from build123d import *

# Parameters (mm, degrees)
SKETCH_W     = 40
SKETCH_H     = 20
PAD_DEPTH    = 2
SKETCH001_W  = 40
SKETCH001_H  = 2.5
PAD001_DEPTH = 10


with BuildPart() as part:
    # Sketch → Pad (new body)
    with BuildSketch(Plane.XY):
        with Locations((20, 10)):
            Rectangle(SKETCH_W, SKETCH_H)
    extrude(amount=PAD_DEPTH)

    # Sketch001 (on Face6 of Pad) → Pad001 (join)
    with BuildSketch(Plane.XY.offset(2)):
        with Locations((20, 1.25)):
            Rectangle(SKETCH001_W, SKETCH001_H)
        with Locations((20, 18.75)):
            Rectangle(SKETCH001_W, SKETCH001_H)
        Polygon((0, 2.5), (0, 0), align=None)
    extrude(amount=PAD001_DEPTH)


solid = part.part
Build history of the part. All positions in model axes, mm. A direction names the side the tool comes from. Round coordinates to 2 decimals unless told otherwise and drop trailing zeros. Write each loop counter-clockwise with the first axis right and the second up, starting at its lowest first coordinate (ties: lowest second). Pieces come first, ordered by that corner, then holes. Notation, with made-up numbers: M -26.75,-8 L 16.25,-8 A17 cw 16.25,-1 Z; hole C -39,-22 d8. An arc over 180 degrees is marked long. Answer as a JSON object with one key per item and string values. Group by question number.
(1) Cut at B-B (x = 29). Give the cut face in (y, z).
(2) Drill centre lines: L1, parallel to Y at x = 37, z = 11; L2, parallel to Z at x = 18.5, y = 8.5. Where is each one in solid material? Low to high.
(3) Cut at A-A (z = 6.5). Give the cut face in (x, y), and give its area (3 significant figures).
(4) Cut at C-C (y = 12.5). Give the cut face in (x, z).
(5) Which spindle directions (+Z, -Z, +X, -X, +Y, -Y) get a long thin tool onto all of the face, cutting with end or side? Do faces 1 (the flat face through (20, 10, 0)), 2 (the flat face through (20, 2.5, 7)). Say none if no direction does.
(6) Mould opens along Y. For faces 3 (the flat face through (20, 17.5, 7)), 4 (the flat face through (20, 1, 12)), 5 (the flat face through (20, 20, 6)) say: pulls with the +Y half, pulls with the -Y half, needs draft (parallel to the pull), parting line crosses it, or undercut.
(7) Flat gauge pin, fed straight in: pin 1 (7.5 mm diameter, centred on x = 28, y = 12.5, fed in from +Z). Where does the tip first touch, or does it go through?
Responses:
{
 "1": {"outline": "M 0,0 L 20,0 L 20,12 L 17.5,12 L 17.5,2 L 2.5,2 L 2.5,12 L 0,12 Z"},
 "2": {"L1": "y = 0 to 2.5, 17.5 to 20", "L2": "z = 0 to 2"},
 "3": {"outline": "M 0,0 L 40,0 L 40,2.5 L 0,2.5 Z; M 0,17.5 L 40,17.5 L 40,20 L 0,20 Z", "area": "200 mm2"},
 "4": {"outline": "M 0,0 L 40,0 L 40,2 L 0,2 Z"},
 "5": {"face 1": "-Z, +X, -X, +Y, -Y", "face 2": "+Z, +X, -X"},
 "6": {"face 3": "undercut", "face 4": "needs draft", "face 5": "pulls with the +Y half"},
 "7": {"pin 1": "stops at z = 2"}
}
